Could you check a few things on this drawing? It's one solid part, dimensions in mm from its lowest x, y, z. A direction names the side the tool comes from. Round coordinates to 2 decimals unless told otherwise and drop trailing zeros. Order: outer loops, then holes, each group sorted by start corner. A loop starts at its lowest first (then second) coordinate and runs counter-clockwise, first axis right, second up.
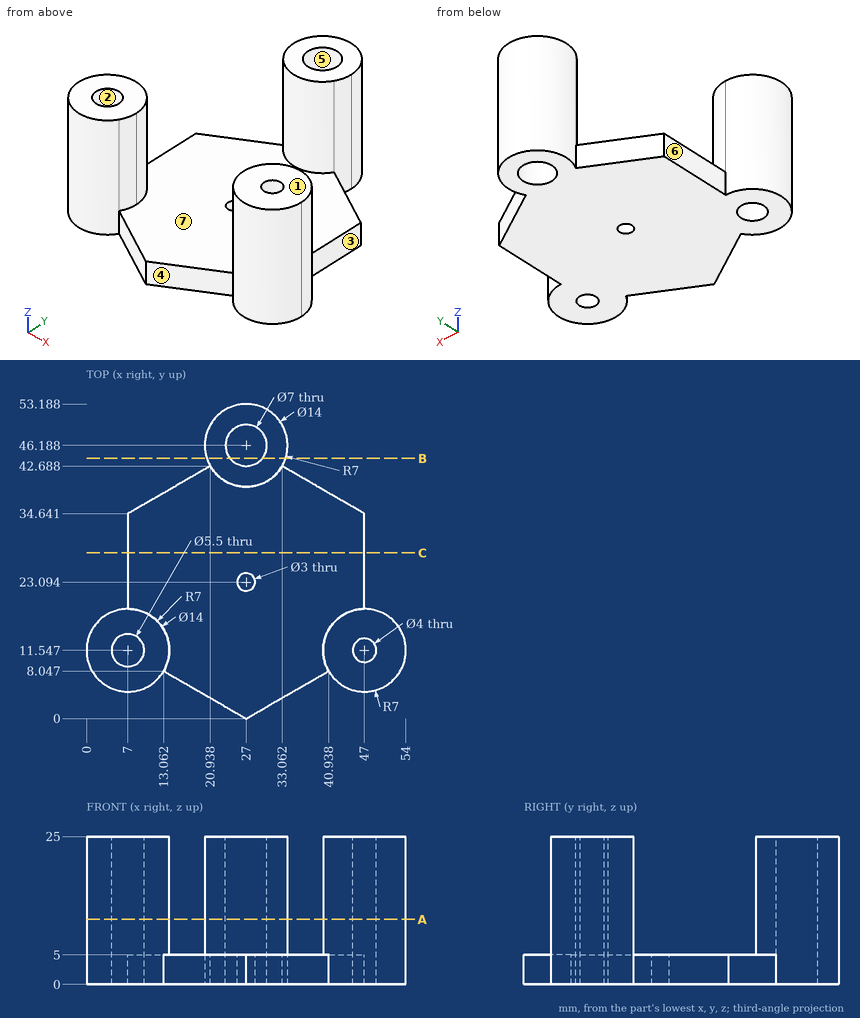
(1) I want a section at C-C, the plane y = 28. List the corners of the cut face in (x, z) for me, plus the area to 3 significant figures.
(2) I'm going to push flat-ended pins straight in: pin 1 Ø1.8 at (x, y) = (27, 23.09) entering from -Z; pin 2 Ø12 at (x, z) = (44, 10.5) entering from +Y; pin 3 Ø3 at (y, z) = (40, 3) entering from +X (1 decimal); pin 4 Ø12 at (x, y) = (46.5, 40) entering from +Z. Where does each tip first touch, or does it pass through?
(3) I want a section at B-B, the plane y = 44. List the corners of the cut face in (x, z) for me, plus the area to 3 significant figures.
(4) I want a section at A-A, the plane z = 11. List the corners of the cut face in (x, y) for me, plus the area to 3 significant figures.
(5) Please list where these lines run through material, in increasing order: probe 1 along X at (y, z) = (46, 14.25) (1 decimal); probe 2 along X at (y, z) = (6.5, 1.75); probe 3 along Z at (x, y) = (42.5, 23).
(6) On a 3-axis mill with a long thin cutter (end or side, diameter ignored), from which of +Z, -Z, +X, -X, +Y, -Y can I reach the whole of each face in a straight line? I mean the marked faces 4, 5, 6 and 7. Say none if no direction works.
(7) If we mould it in two halves opening along X, with no side actions, what happens to the marked faces 1, 2 and 3? For each: pulls with the +X half, pulls with the -X half, needs draft (parallel to the pull), parting line crosses it, or undercut.
Ans:
1. outline: (7, 0) - (47, 0) - (47, 5) - (7, 5) - close
1. area: 200 mm2
2. pin 1: passes through
2. pin 2: stops at y = 37.76
2. pin 3: stops at x = 40.3
2. pin 4: stops at z = 5
3. outline: (20.35, 0) - (24.27, 0) - (24.27, 25) - (20.35, 25) - close; (29.73, 0) - (33.65, 0) - (33.65, 25) - (29.73, 25) - close
3. area: 196 mm2
4. outline: circle Ø14 at (7, 11.55); circle Ø14 at (27, 46.19); circle Ø14 at (47, 11.55); hole circle Ø5.5 at (7, 11.55); hole circle Ø7 at (27, 46.19); hole circle Ø4 at (47, 11.55)
4. area: 387 mm2
5. probe 1: x = 20 to 23.5, 30.5 to 34
5. probe 2: x = 2.15 to 11.85, 15.74 to 38.26, 42.15 to 51.85
5. probe 3: z = 0 to 5
6. face 4: +Z, -Z, -Y
6. face 5: +Z, -Z
6. face 6: +Z, -Z, -X, +Y
6. face 7: +Z
7. face 1: needs draft
7. face 2: undercut
7. face 3: pulls with the +X half
